Source: CAD feature listing. Evaluate the final solid. Frame: model axes, mm. Face numbers are marked on the shaded views. A direction names the side the tool comes from. Round coordinates to 2 decimals unless told otherwise and drop trailing zeros. Write each loop counter-clockwise with the first axis right and the second up, starting at its lowest first coordinate (ties: lowest second). Pieces come first, ordered by that corner, then holes.
```python
from build123d import *

# Parameters (mm, degrees)
F1_DEPTH = 24
F3_D     = 3
F4_R     = 0.5


with BuildPart() as f1:
    # F0 (on Right) → F1 (new body)
    with BuildSketch(Plane.YZ):
        Polygon((-3.25, 5), (-4.75, 5), (-4.75, 0), (4.75, 0), (4.75, 5), (3.25, 5), (3.25, 2.5), (-3.25, 2.5), align=None)
    extrude(amount=F1_DEPTH)

    # F3 (through all)
    with Locations(Plane.XY.offset(2.5)):
        with Locations((12, 0)):
            Hole(F3_D / 2)

    # F4
    f4_edges = [f1.edges().sort_by_distance(p)[0] for p in [
        (12, 3.25, 5),
        (12, -3.25, 5),
        (12, -4.75, 5),
        (12, 4.75, 5),
        (0, 4, 5),
        (0, -4, 5),
        (24, -4, 5),
        (24, 4, 5),
    ]]
    fillet(f4_edges, radius=F4_R)


solid = f1.part
```
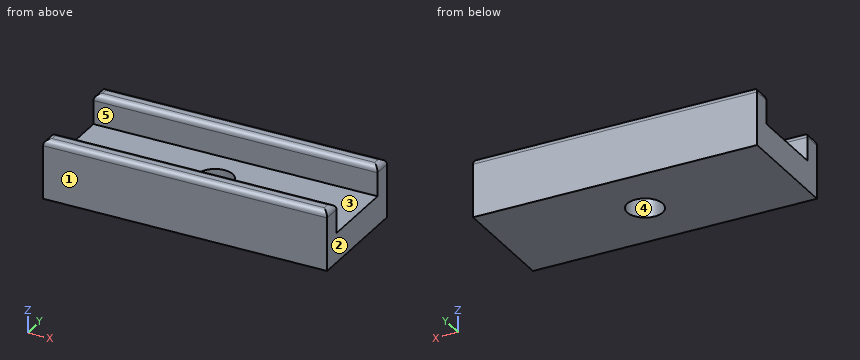
Q1. Set-up query: the marked faces 4 and 5. Return all of +Z, -Z, +X, -X, +Y, -Y with unobstructed straight access to the full face (end or side cutting, diameter ignored); none if empty.
Q2. Section query C-C, the plane y = 0. Output: boundary loops of the cut face in (x, z), and give its area (3 significant figures).
Q3. Line query: line 1 (Y direction, x = 12, z = 1.45); line 2 (Z direction, x = 6.75, y = 0.25); line 3 (X direction, y = 0.25, z = 2.05). Output: solid intervals per line, ascending.
Q4. Section query B-B, the plane z = 2.8. Output: boundary loops of the cut face in (x, y), and give its area (3 significant figures).
Q5. Section query D-D, the plane x = 21.75. Output: boundary loops of the cut face in (y, z).
Q6. Section query A-A, the plane x = 12. Output: boundary loops of the cut face in (y, z), and give its area (3 significant figures).
Q7. Mould query, pull axis Y, two halves, no side actions, for the marked faces 1, 2 and 3. Classes: pulls with the +Y half, pulls with the -Y half, needs draft (parallel to the pull), parting line crosses it, or undercut.
Q8. Pin query (flat end, axial travel): P1, Ø5, axis at x = 12, y = 0, coming from the +Z side; P2, Ø4, axis at x = 16, y = -1.5, coming from the -Z side. Return the tip coordinate at first contact, or that it passes through.
Filled in:
1. face 4: +Z, -Z
1. face 5: +Z, +X, -X
2. outline: (0, 0) - (10.5, 0) - (10.5, 2.5) - (0, 2.5) - close; (13.5, 0) - (24, 0) - (24, 2.5) - (13.5, 2.5) - close
2. area: 52.5 mm2
3. line 1: y = -4.75 to -1.5, 1.5 to 4.75
3. line 2: z = 0 to 2.5
3. line 3: x = 0 to 10.52, 13.48 to 24
4. outline: (0, -4.75) - (24, -4.75) - (24, -3.25) - (0, -3.25) - close; (0, 3.25) - (24, 3.25) - (24, 4.75) - (0, 4.75) - close
4. area: 72.0 mm2
5. outline: (-4.75, 0) - (4.75, 0) - (4.75, 4.5) arc R0.5 ccw to (4.25, 5) - (3.75, 5) arc R0.5 ccw to (3.25, 4.5) - (3.25, 2.5) - (-3.25, 2.5) - (-3.25, 4.5) arc R0.5 ccw to (-3.75, 5) - (-4.25, 5) arc R0.5 ccw to (-4.75, 4.5) - close
6. outline: (-4.75, 0) - (-1.5, 0) - (-1.5, 2.5) - (-3.25, 2.5) - (-3.25, 4.5) arc R0.5 ccw to (-3.75, 5) - (-4.25, 5) arc R0.5 ccw to (-4.75, 4.5) - close; (1.5, 0) - (4.75, 0) - (4.75, 4.5) arc R0.5 ccw to (4.25, 5) - (3.75, 5) arc R0.5 ccw to (3.25, 4.5) - (3.25, 2.5) - (1.5, 2.5) - close
6. area: 23.5 mm2
7. face 1: pulls with the -Y half
7. face 2: needs draft
7. face 3: undercut
8. P1: stops at z = 2.5
8. P2: stops at z = 0
